from build123d import *

# Parameters (mm, degrees)
F1_DEPTH = 25.4


with BuildPart() as f1:
    # F0 (on Front) → F1 (new body)
    with BuildSketch(Plane.XZ):
        with BuildLine():
            ThreePointArc((1.8673827959, 32.4323775117), (23.2426437423, 24.7104189311), (36.799872741, 42.9513609771))
            ThreePointArc((36.799872741, 42.9513609771), (19.7876276974, 61.892059347), (-0.8641750005, 47.0034871694))
            Line((-0.8641750005, 47.0034871694), (0, 47.0034871694))
            Line((0, 47.0034871694), (0, 36.0343878183))
            ThreePointArc((0, 36.0343878183), (0.8375229775, 34.1835262685), (1.8673827959, 32.4323775117))
        make_face()
        with BuildLine():
            Line((0, 47.0034871694), (-0.8641750005, 47.0034871694))
            ThreePointArc((-0.8641750005, 47.0034871694), (-1.2412821306, 41.4551869754), (0, 36.0343878183))
            Line((0, 36.0343878183), (0, 47.0034871694))
        make_face()
        with BuildLine():
            ThreePointArc((0, 36.0343878183), (-1.2412821306, 41.4551869754), (-0.8641750005, 47.0034871694))
            Line((-0.8641750005, 47.0034871694), (-23.2337535647, 47.0034871694))
            Line((-23.2337535647, 47.0034871694), (-23.2337535647, 22.2208360441))
            ThreePointArc((-23.2337535647, 22.2208360441), (-21.4104164375, 20.2400678606), (-19.8069730457, 18.0774374795))
            Line((-19.8069730457, 18.0774374795), (0, 31.1956086661))
            Line((0, 31.1956086661), (0, 36.0343878183))
        make_face()
        with BuildLine():
            Line((0, 31.1956086661), (1.8673827959, 32.4323775117))
            ThreePointArc((1.8673827959, 32.4323775117), (0.8375229775, 34.1835262685), (0, 36.0343878183))
            Line((0, 36.0343878183), (0, 31.1956086661))
        make_face()
        with BuildLine():
            Line((0, 0), (0, 31.1956086661))
            Line((0, 31.1956086661), (-19.8069730457, 18.0774374795))
            ThreePointArc((-19.8069730457, 18.0774374795), (-16.6623702443, 11.3758208608), (-15.5836263057, 4.0521261923))
            ThreePointArc((-15.5836263057, 4.0521261923), (-15.6650834504, 2.0195446596), (-15.9089324228, 0))
            Line((-15.9089324228, 0), (0, 0))
        make_face()
        with BuildLine():
            Line((-23.2337535647, 15.8078785033), (-23.2337535647, 22.2208360441))
            ThreePointArc((-23.2337535647, 22.2208360441), (-65.1067949461, -3.8997751366), (-15.9089324228, 0))
            Line((-15.9089324228, 0), (-23.2337535647, 0))
            Line((-23.2337535647, 0), (-23.2337535647, 15.8078785033))
        make_face()
        with BuildLine():
            ThreePointArc((-19.8069730457, 18.0774374795), (-21.4104164375, 20.2400678606), (-23.2337535647, 22.2208360441))
            Line((-23.2337535647, 22.2208360441), (-23.2337535647, 15.8078785033))
            Line((-23.2337535647, 15.8078785033), (-19.8069730457, 18.0774374795))
        make_face()
        with BuildLine():
            ThreePointArc((-15.5836263057, 4.0521261923), (-16.6623702443, 11.3758208608), (-19.8069730457, 18.0774374795))
            Line((-19.8069730457, 18.0774374795), (-23.2337535647, 15.8078785033))
            Line((-23.2337535647, 15.8078785033), (-23.2337535647, 0))
            Line((-23.2337535647, 0), (-15.9089324228, 0))
            ThreePointArc((-15.9089324228, 0), (-15.6650834504, 2.0195446596), (-15.5836263057, 4.0521261923))
        make_face()
    extrude(amount=F1_DEPTH)


solid = f1.part
Part model, mm, in its own coordinate system. A direction names the side the tool comes from. Coordinates: 2 decimals unless noted, no trailing zeros. Order: outer loops, then holes, each group sorted by start corner. A loop starts at its lowest first (then second) coordinate and runs counter-clockwise, first axis right, second up. Notation, with made-up numbers: M 69,58 L 75,58 A14 ccw 75,63 Z; hole C 32.25,2 d10. An arc over 180 degrees is marked long. Use a Markdown table: item, result.
(1) Tool access for faces 3 (the flat face through (0, -13, 15)), 4 (the flat face through (-12, -13, 47.003)), 5 (the flat face through (-8, -13, 0)): list every direction of +Z, -Z, +X, -X, +Y, -Y with a clear straight run to the whole face (end or side of a thin tool).
A:
| item | result |
|---|---|
| face 3 | -Z, +Y, -Y |
| face 4 | +Z, -X, +Y, -Y |
| face 5 | -Z, +X, +Y, -Y |
(2) Pull direction X, two halves, no side cores. Call faces 1 (the flat face through (-16, 0, 21)), 2 (the flat face through (-23.234, -13, 35)): released by +X, released by -X, zero draft, split by the parting line, or undercut.
A:
| item | result |
|---|---|
| face 1 | zero draft |
| face 2 | undercut |
(3) Cut at C-C on z = -15. Write the cut outline in (x, y), then the cut area to 3 significant figures.
A:
| item | result |
|---|---|
| outline | M -57.78,-25.4 L -24.19,-25.4 L -24.19,0 L -57.78,0 Z |
| area | 853 mm^2 |
(4) Cut at A-A on y = -4.25. Write the cut outline in (x, z).
A:
| item | result |
|---|---|
| outline | M -23.23,22.22 A25.4 ccw long -15.91,0 L 0,0 L 0,31.2 L 1.87,32.43 A19.05 ccw long -0.86,47 L -23.23,47 Z |
(5) Flat gauge pins, fed straight in: pin 1 (4 mm diameter, centred on x = -28.5, z = 30.5, fed in from -Y); pin 2 (6.5 mm diameter, centred on x = -16.5, y = -15.5, fed in from +Z); pin 3 (12.5 mm diameter, centred on x = -7.5, y = -14, fed in from -Z); pin 4 (10 mm diameter, centred on x = 20, y = -22.5, fed in from -Z). Where does each tip first touch, or does it go through?
A:
| item | result |
|---|---|
| pin 1 | passes through |
| pin 2 | stops at z = 47 |
| pin 3 | stops at z = 0 |
| pin 4 | stops at z = 23.9 |
(6) Probe L1, parallel to X at y = -19, z = 26; L2, parallel to Z at x = -1.5, y = -2; L3, parallel to Z at x = -40, y = -7.25. List the from-to ranges inside material, lowest first.
A:
| item | result |
|---|---|
| L1 | x = -53.77 to -28.2, -23.23 to 0, 9.06 to 26.44 |
| L2 | z = 0 to 47 |
| L3 | z = -21.33 to 29.43 |
(7) Cut at B-B on x = -9. Write the cut outline in (y, z).
A:
| item | result |
|---|---|
| outline | M -25.4,0 L 0,0 L 0,47 L -25.4,47 Z |
